from build123d import *

# Parameters (mm, degrees)
CROQUIS1_W              = 22
CROQUIS1_H              = 50
SALIENTE_EXTRUIR2_DEPTH = 3
CROQUIS2_W              = 27
CROQUIS2_H              = 22
SALIENTE_EXTRUIR3_DEPTH = 3
CROQUIS3_W              = 3
CROQUIS3_H              = 22
SALIENTE_EXTRUIR4_DEPTH = 50
CROQUIS4_W              = 10
CROQUIS4_H              = 22
CROQUIS4_R              = 1.5
SALIENTE_EXTRUIR5_DEPTH = 3
REDONDEO1_R             = 2


with BuildPart() as part:
    # Croquis1 → Saliente-Extruir2 (new body)
    with BuildSketch(Plane(origin=(0, 0, 0), x_dir=(0, 0, -1), z_dir=(1, 0, 0))):
        with Locations((-11, -25)):
            Rectangle(CROQUIS1_W, CROQUIS1_H)
    extrude(amount=SALIENTE_EXTRUIR2_DEPTH)

    # Croquis2 → Saliente-Extruir3 (add)
    with BuildSketch(Plane(origin=(0, -50, 0), x_dir=(-1, 0, 0), z_dir=(0, -1, 0))):
        with Locations((-13.5, -11)):
            Rectangle(CROQUIS2_W, CROQUIS2_H)
    extrude(amount=SALIENTE_EXTRUIR3_DEPTH)

    # Croquis3 → Saliente-Extruir4 (add)
    with BuildSketch(Plane(origin=(0, -50, 0), x_dir=(1, 0, 0), z_dir=(0, 1, 0))):
        with Locations((25.5, -11)):
            Rectangle(CROQUIS3_W, CROQUIS3_H)
    extrude(amount=SALIENTE_EXTRUIR4_DEPTH)

    # Croquis4 → Saliente-Extruir5 (add)
    # profile 1 of 2: a face of its own
    with BuildSketch(Plane(origin=(0, 0, 0), x_dir=(1, 0, 0), z_dir=(0, 1, 0))):
        with Locations((-2, -11)):
            Rectangle(CROQUIS4_W, CROQUIS4_H)
        with Locations(Location((-3, -4, 0), (0, 0, 270))):
            Circle(CROQUIS4_R, mode=Mode.SUBTRACT)
        with Locations(Location((-3, -18, 0), (0, 0, 270))):
            Circle(CROQUIS4_R, mode=Mode.SUBTRACT)
    # profile 2 of 2: a face of its own
    with BuildSketch(Plane(origin=(0, 0, 0), x_dir=(1, 0, 0), z_dir=(0, 1, 0))):
        with Locations((29, -11)):
            Rectangle(CROQUIS4_W, CROQUIS4_H)
        with Locations(Location((30, -18, 0), (0, 0, 270))):
            Circle(CROQUIS4_R, mode=Mode.SUBTRACT)
        with Locations(Location((30, -4, 0), (0, 0, 270))):
            Circle(CROQUIS4_R, mode=Mode.SUBTRACT)
    extrude(amount=SALIENTE_EXTRUIR5_DEPTH)

    # Redondeo1
    redondeo1_edges = [part.edges().sort_by_distance(p)[0] for p in [
        (27, -26.5, 0),
        (27, -26.5, 22),
        (27, -53, 11),
        (13.5, -53, 22),
        (0, -53, 11),
        (13.5, -53, 0),
        (-3.5, 0, 0),
        (-7, 0, 11),
        (-3.5, 0, 22),
        (0, -26.5, 0),
        (0, -26.5, 22),
        (30.5, 0, 22),
        (34, 0, 11),
        (30.5, 0, 0),
    ]]
    fillet(redondeo1_edges, radius=REDONDEO1_R)


solid = part.part
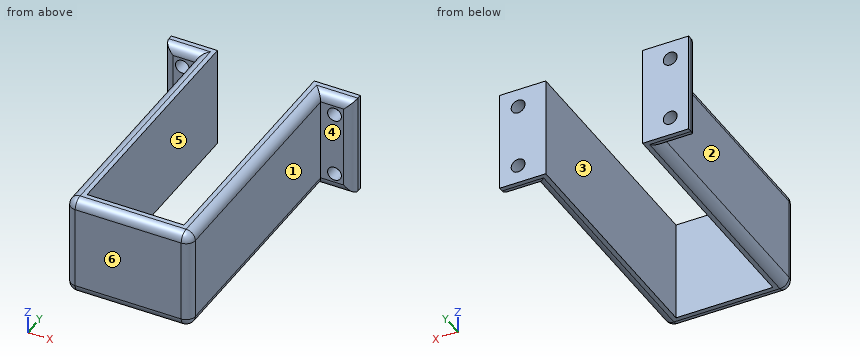
Read the model definition and answer for the solid it produces. Units are mm, in the model's axes. Face numbers are marked on the shaded views. A direction names the side the tool comes from. Coordinates: 2 decimals unless noted, no trailing zeros. Loops run counter-clockwise (first coordinate to the right, second up) from the corner with the lowest first, then second, coordinate; pieces in that order, holes last.
Q1. The part is cut by section B-B on x = 30. Write down the section's boundary in (y, z), and give its area (3 significant figures).
Q2. The part is cut by section C-C on z = 18. Write down the section's boundary in (x, y), and give its area (3 significant figures).
Q3. Each of these flat-tipped pins is pushed along its axis until it touches: pin 1 Ø12 at (x, z) = (6, 12) entering from +Y; pin 2 Ø5 at (x, y) = (6.5, -3.5) entering from -Z; pin 3 Ø5.5 at (x, z) = (-1.5, 15.5) entering from -Y; pin 4 Ø9 at (y, z) = (-17.5, 10.5) entering from +X. Where does it stop, or does it pass through?
Q4. Which of the six approach directions +Z, -Z, +X, -X, +Y, -Y give full straight-line access (tool end or side, diameter ignored) to the marked faces 4, 5 and 6?
Q5. The part is cut by section D-D on x = 11.5. Write down the section's boundary in (y, z).
Q6. The part is cut by section A-A on y = -40.5. Write down the section's boundary in (x, z), and give its area (3 significant figures).
Q7. The mould has two halves that part along X. Classify the marked faces 1, 2 and 3: +X half, -X half, draft (parallel to the pull), parting line (faces both ways), or undercut.
Q8. Consider probe 1 along X at (y, z) = (2.4, 4); probe 2 along X at (y, z) = (-2, 13.75); probe 3 along X at (y, z) = (1.05, 4). Determine where each line is inside the solid, lowest interval first.
Results below:
1. outline: (0, 2) arc R2 ccw to (2, 0) - (3, 0) - (3, 2.5) - (0, 2.5) - close; (0, 5.5) - (3, 5.5) - (3, 16.5) - (0, 16.5) - close; (0, 19.5) - (3, 19.5) - (3, 22) - (2, 22) arc R2 ccw to (0, 20) - close
1. area: 46.3 mm2
2. outline: (-7, 2) arc R2 ccw to (-5, 0) - (-4.5, 0) - (-4.5, 3) - (-7, 3) - close; (-1.5, 0) - (0, 0) - (0, -51) arc R2 ccw to (2, -53) - (25, -53) arc R2 ccw to (27, -51) - (27, 0) - (28.5, 0) - (28.5, 3) - (24, 3) - (24, -50) - (3, -50) - (3, 3) - (-1.5, 3) - close; (31.5, 0) - (32, 0) arc R2 ccw to (34, 2) - (34, 3) - (31.5, 3) - close
2. area: 420 mm2
3. pin 1: stops at y = 3
3. pin 2: passes through
3. pin 3: stops at y = -52.85
3. pin 4: stops at x = 27
4. face 4: +Z, -Z, +X, -Y
4. face 5: +Z, -Z, +Y
4. face 6: +Z, -Z, +X, -X, -Y
5. outline: (-53, 2) arc R2 ccw to (-51, 0) - (-50, 0) - (-50, 22) - (-51, 22) arc R2 ccw to (-53, 20) - close
6. outline: (0, 2) arc R2 ccw to (2, 0) - (3, 0) - (3, 22) - (2, 22) arc R2 ccw to (0, 20) - close; (24, 0) - (25, 0) arc R2 ccw to (27, 2) - (27, 20) arc R2 ccw to (25, 22) - (24, 22) - close
6. area: 129 mm2
7. face 1: +X half
7. face 2: -X half
7. face 3: undercut
8. probe 1: x = -7 to -4.5, -1.5 to 3, 24 to 28.5, 31.5 to 34
8. probe 2: x = 0 to 3, 24 to 27
8. probe 3: x = -6.76 to -4.5, -1.5 to 3, 24 to 28.5, 31.5 to 33.76
